Here's how the part is built. I have some questions about the finished solid (model axes, mm). Face numbers are marked on the shaded views. Give positions to 0.01 mm unless a question says otherwise; leave off trailing zeros. Write each loop counter-clockwise with the first axis right and the second up, starting at its lowest first coordinate (ties: lowest second). Pieces come first, ordered by that corner, then holes. Notation, with made-up numbers: (-26, 38.5) - (-10, 38.5) arc R28 cw to (-10, 64.5) - close; hole circle Ø4 at (68.5, 17). An arc over 180 degrees is marked (long way). Write each question's results on one line, items separated by ' | '. Start each with the question number.
Item 1: Suppose I cut it at C-C on z = 9.5. List the corners of the cut face in (x, y) for me, then the cut area to 3 significant figures.
Item 2: Please list where these lines run through material, in increasing order: line 1 along Z through (x, y) = (7, -2.25); line 2 along Z through (x, y) = (4.5, -4); line 3 along X through (y, z) = (-4.5, 17.5).
Item 3: Suppose I cut it at D-D on y = -4.5. List the corners of the cut face in (x, z) for me (3 decimals), then the cut area to 3 significant figures.
Item 4: Suppose I cut it at B-B on x = 8.5. List the corners of the cut face in (y, z) for me.
Item 5: We'd pull the mould along X, two halves only. Please class the marked faces 1, 2 and 3: +X half, -X half, draft (parallel to the pull), parting line (faces both ways), or undercut.
Item 6: Suppose I cut it at A-A on y = -5.5. List the corners of the cut face in (x, z) for me (3 decimals).
Item 7: Will these pins go through, and if not, where does the flat tip stop? P1, Ø2, axis at y = -2, z = 14.5, coming from the +X side; P2, Ø4, axis at y = -6, z = 17, coming from the -X side; P3, Ø2, axis at y = -3.5, z = 11, coming from the +X side.
Autodesk Inventor part; units mm, degrees
ref_plane "YZ Plane" through (0, 0, 0) normal (1, 0, 0) x (0, 1, 0)
ref_plane "XZ Plane" through (0, 0, 0) normal (0, 1, 0) x (-1, 0, 0)
ref_plane "XY Plane" through (0, 0, 0) normal (0, 0, 1) x (1, 0, 0)
sketch "Boceto1" plane through (0, 0, 0) normal (0, 0, 1) x (1, 0, 0)
  line L0 (0.1921, 0) -> (13.6079, 0)
  line L1 (0.1102, -0.1574) -> (4.514, -6.4466)
  line L2 (0, 0) -> (7.6778, 0) construction
  line L3 (6.1507, -7.2995) -> (6.8282, -7.3)
  arc A0 (0.1921, 0) -> (0.1102, -0.1574) centre (0.1921, -0.1) ccw
  arc A1 (13.6898, -0.1574) -> (13.6079, 0) centre (13.6079, -0.1) ccw
  line L4 (6.8282, 0) -> (6.8282, -7.3)
  line L5 (13.6898, -0.1574) -> (9.144, -6.4684)
  line L6 (7.5227, -7.2995) -> (6.8282, -7.3)
  arc A2 (7.5227, -7.2995) -> (9.144, -6.4684) centre (7.5211, -5.2995) ccw
  arc A3 (4.514, -6.4466) -> (6.1507, -7.2995) centre (6.1523, -5.2995) ccw
  point P0 (13.8, 0)
  point P1 (5.1106, -7.2986)
  point P2 (8.5459, -7.2986)
  dimension "d7" = 13.8
  dimension "d9" = 8.91
  dimension "d10" = 55
  dimension "d11" = 0.1
  dimension "d14" = 2
  dimension "d15" = 7.3
extrude "Extrusión1" add sketch "Boceto1" along normal blind 23
sketch "Boceto2" plane through (0.1921, 0, 0) normal (0, 1, 0) x (1, 0, 0)
  circle A0 centre (6.6362, -17.5) radius 3.375
  point P0 (-0.1921, 0)
  point P1 (6.6362, -23)
  dimension "d17" = 6.75
extrude "Extrusión2" cut sketch "Boceto2" against normal blind 7.3
properties part number "Tuerca" material "Acero, galvanizado"
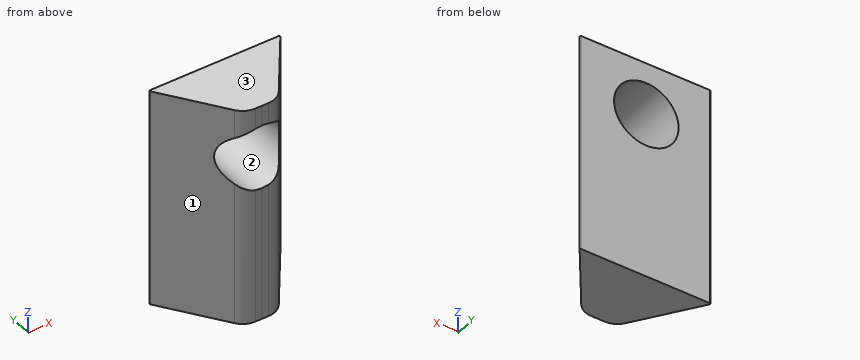
Checked values:
1) outline: (0.11, -0.16) - (4.51, -6.45) arc R2 ccw to (6.15, -7.3) - (6.83, -7.3) - (7.52, -7.3) arc R2 ccw to (9.14, -6.47) - (13.69, -0.16) arc R0.1 ccw to (13.61, 0) - (0.19, 0) arc R0.1 ccw to start | area: 62.6 mm^2
2) line 1: z = 0 to 14.13, 20.87 to 23 | line 2: z = 0 to 15.06, 19.94 to 23 | line 3: x = 3.15 to 3.45, 10.2 to 10.56
3) outline: (3.151, 0) - (10.562, 0) - (10.562, 23) - (3.151, 23) - close; hole circle Ø6.75 at (6.828, 17.5) | area: 135 mm^2
4) outline: (-7.04, 0) - (0, 0) - (0, 14.57) - (-7.04, 14.57) - close; (-7.04, 20.43) - (0, 20.43) - (0, 23) - (-7.04, 23) - close
5) face 1: -X half | face 2: undercut | face 3: draft
6) outline: (3.851, 0) - (9.842, 0) - (9.842, 15.98) arc R3.375 cw to (3.851, 15.91) - close; (3.851, 19.09) arc R3.375 cw to (9.842, 19.02) - (9.842, 23) - (3.851, 23) - close
7) P1: stops at x = 13.08 | P2: stops at x = 2.8 | P3: stops at x = 12
